Autodesk Inventor part; units mm, degrees
ref_plane "YZ Plane" through (0, 0, 0) normal (1, 0, 0) x (0, 1, 0)
ref_plane "XZ Plane" through (0, 0, 0) normal (0, 1, 0) x (-1, 0, 0)
ref_plane "XY Plane" through (0, 0, 0) normal (0, 0, 1) x (1, 0, 0)
sketch "Boceto1" plane through (0, 0, 0) normal (1, 0, 0) x (0, 1, 0)
  line L0 (8, 0) -> (8, -3)
  line L1 (8, -3) -> (-8, -3)
  line L2 (-8, -3) -> (-8, 0)
  line L3 (8, 0) -> (-8, 0)
  line L4 (-18.175, -6.5) -> (11.175, -6.5)
  line L5 (1.5, 3) -> (1.5, 10)
  line L6 (1.5, 10) -> (-1.5, 10)
  line L7 (-1.5, 10) -> (-1.5, 3)
  line L8 (-1.5, 3) -> (1.5, 3)
  line L9 (-9.5, 39) -> (2.5, 39)
  line L10 (2.5, 39) -> (2.5, 16)
  line L11 (-9.5, 39) -> (-9.5, 16)
  line L12 (-9.5, 16) -> (2.5, 16)
  circle A0 centre (-3.5, 41.5) radius 1.5
  circle A1 centre (-3.5, 13.5) radius 1.5
  line L13 (11.175, -6.5) -> (11.175, 45.5)
  line L14 (-18.175, 45.5) -> (-18.175, -6.5)
  line L15 (2.5, 23.4783) -> (2.5, 27.5)
  line L16 (6.175, 50.5) -> (1.5, 50.5)
  line L17 (-8.5, 50.5) -> (-13.175, 50.5)
  line L18 (1.5, 50.5) -> (-8.5, 50.5)
  arc A2 (-13.175, 50.5) -> (-18.175, 45.5) centre (-13.175, 45.5) ccw
  arc A3 (11.175, 45.5) -> (6.175, 50.5) centre (6.175, 45.5) ccw
  point P0 (11.175, 50.5)
  point P1 (-18.175, 50.5)
  dimension "d28" = 5
extrude "Extrusión1" add sketch "Boceto1" along normal blind 3
properties part number "muñeca5"
Check sheet for the modelled part. Datum: model origin and axes. Units: mm. A direction names the side the tool comes from. Give positions to 0.01 mm unless a question says otherwise; leave off trailing zeros. Loops run counter-clockwise (first coordinate to the right, second up) from the corner with the lowest first, then second, coordinate; pieces in that order, holes last. Notation, with made-up numbers: M 38.25,51.25 L 75.25,51.25 A25 cw 75.25,82.25 Z; hole C 2.5,50.5 d3. An arc over 180 degrees is marked long. Use a Markdown table: item, result. Add a question column.
Q1. Mould release check, pull along Z, two halves, no side actions. Record for faces 3 (the flat face through (1, -4, -6.5)), 4 (the cylindrical face through (1.479, -2.114, 14.075)), 5 (the flat face through (1, 11.175, 19)), 6 (the flat face through (1, 1.5, 6)): pulls with the +Z half, pulls with the -Z half, needs draft (parallel to the pull), parting line crosses it, or undercut.
Q2. Sectioned sample at A-A, the plane z = 41.5. Record the cut outline in (x, y) (3 decimals).
Q3. Sectioned sample at C-C, the plane y = -6.5. Record the cut outline in (x, z).
Q4. Sectioned sample at D-D, the plane y = -3.5. Record the cut outline in (x, z).
Q5. Sectioned sample at B-B, the plane x = 2.45. Record the cut outline in (y, z) (3 decimals), then the cut area to 3 significant figures.
Q6. Scan lines: line 1 along Z through (x, y) = (2.2, -3.5); line 2 along Z through (x, y) = (1.15, 1.25); line 3 along Z through (x, y) = (1.3, -4). Record each from-to range of solid material in increasing order. Write a range as [from, to].
Q7. Tool access check on faces 1 (the flat face through (1, -4, 16)), 2 (the flat face through (0, -10, 22)). Record the directions out of +Z, -Z, +X, -X, +Y, -Y that give a thin tool (end or side, any length) a straight path to the whole face; none if there is none.
Verdict:
| question | item | result |
|---|---|---|
| 1 | face 3 | pulls with the -Z half |
| 1 | face 4 | undercut |
| 1 | face 5 | needs draft |
| 1 | face 6 | undercut |
| 2 | outline | M 0,-18.175 L 3,-18.175 L 3,-5 L 0,-5 Z; M 0,-2 L 3,-2 L 3,11.175 L 0,11.175 Z |
| 3 | outline | M 0,-6.5 L 3,-6.5 L 3,-3 L 0,-3 Z; M 0,0 L 3,0 L 3,16 L 0,16 Z; M 0,39 L 3,39 L 3,50.5 L 0,50.5 Z |
| 4 | outline | M 0,-6.5 L 3,-6.5 L 3,-3 L 0,-3 Z; M 0,0 L 3,0 L 3,12 L 0,12 Z; M 0,15 L 3,15 L 3,16 L 0,16 Z; M 0,39 L 3,39 L 3,40 L 0,40 Z; M 0,43 L 3,43 L 3,50.5 L 0,50.5 Z |
| 5 | outline | M -18.175,-6.5 L 11.175,-6.5 L 11.175,45.5 A5 ccw 6.175,50.5 L -13.175,50.5 A5 ccw -18.175,45.5 Z; hole M -9.5,16 L 2.5,16 L 2.5,39 L -9.5,39 Z; hole M -8,-3 L 8,-3 L 8,0 L -8,0 Z; hole C -3.5,13.5 d3; hole C -3.5,41.5 d3; hole M -1.5,3 L 1.5,3 L 1.5,10 L -1.5,10 Z |
| 5 | area | 1,300 mm^2 |
| 6 | line 1 | [-6.5, -3], [0, 12], [15, 16], [39, 40], [43, 50.5] |
| 6 | line 2 | [-6.5, -3], [0, 3], [10, 16], [39, 50.5] |
| 6 | line 3 | [-6.5, -3], [0, 12.09], [14.91, 16], [39, 40.09], [42.91, 50.5] |
| 7 | face 1 | +X, -X |
| 7 | face 2 | +Z, -Z, -X, +Y, -Y |
